Could you check a few things on this model? Use its own coordinates, in mm. Round coordinates to 2 decimals unless told otherwise and drop trailing zeros. Order: outer loops, then holes, each group sorted by start corner. A loop starts at its lowest first (then second) coordinate and runs counter-clockwise, first axis right, second up. Notation, with made-up numbers: M 41.5,-23 L 53.5,-23 A31 ccw 53.5,7 Z; hole C 54,37.5 d5. An arc over 180 degrees is marked long. Write each question's results on one line, items separated by ' | '. Start each with the question number.
1. Suppose I cut it at C-C on z = 1.25. Write out the boundary of the cut face in (x, y), and give its area (3 significant figures).
2. Suppose I cut it at B-B on x = 7. Write out the boundary of the cut face in (y, z), and give its area (3 significant figures).
3. I'm going to push a flat-ended pin straight in: pin 1 (1.8 mm diameter, centred on x = -7, y = 42, fed in from +Z). Where does the tip first touch, or does it pass through?
4. Suppose I cut it at D-D on x = -6.5. Write out the boundary of the cut face in (y, z), and give its area (3 significant figures).
5. Suppose I cut it at A-A on y = 42. Write out the boundary of the cut face in (x, z).
6. Please list where these lines run through material, in increasing order: L1, parallel to Y at x = 7, z = 1.15; L2, parallel to Y at x = -6.5, z = 1.3; L3, parallel to Y at x = -3.25, z = 0.25.
from build123d import *

# Parameters (mm, degrees)
IZIM1_R                     = 1.5
Y_KSEKLIK_EKSTR_ZYON1_DEPTH = 1.6


with BuildPart() as part:
    # Çizim1 → Yükseklik-Ekstrüzyon1 (new body)
    with BuildSketch(Plane.XY):
        Polygon((0, -55), (-10, -45), (-10, 45), (10, 45), (10, -45), align=None)
        with Locations((-7, 42)):
            Circle(IZIM1_R, mode=Mode.SUBTRACT)
        with Locations((7, 42)):
            Circle(IZIM1_R, mode=Mode.SUBTRACT)
    extrude(amount=Y_KSEKLIK_EKSTR_ZYON1_DEPTH)


solid = part.part
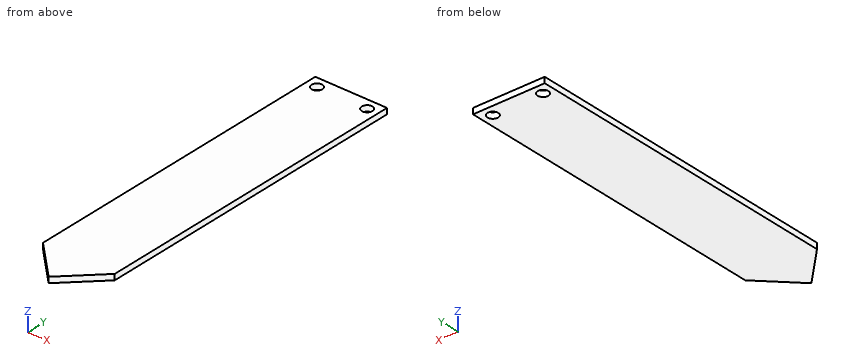
Filled sheet:
1) outline: M -10,-45 L 0,-55 L 10,-45 L 10,45 L -10,45 Z; hole C -7,42 d3; hole C 7,42 d3 | area: 1,890 mm^2
2) outline: M -48,0 L 40.5,0 L 40.5,1.6 L -48,1.6 Z; M 43.5,0 L 45,0 L 45,1.6 L 43.5,1.6 Z | area: 144 mm^2
3) pin 1: passes through
4) outline: M -48.5,0 L 40.59,0 L 40.59,1.6 L -48.5,1.6 Z; M 43.41,0 L 45,0 L 45,1.6 L 43.41,1.6 Z | area: 145 mm^2
5) outline: M -10,0 L -8.5,0 L -8.5,1.6 L -10,1.6 Z; M -5.5,0 L 5.5,0 L 5.5,1.6 L -5.5,1.6 Z; M 8.5,0 L 10,0 L 10,1.6 L 8.5,1.6 Z
6) L1: y = -48 to 40.5, 43.5 to 45 | L2: y = -48.5 to 40.59, 43.41 to 45 | L3: y = -51.75 to 45
